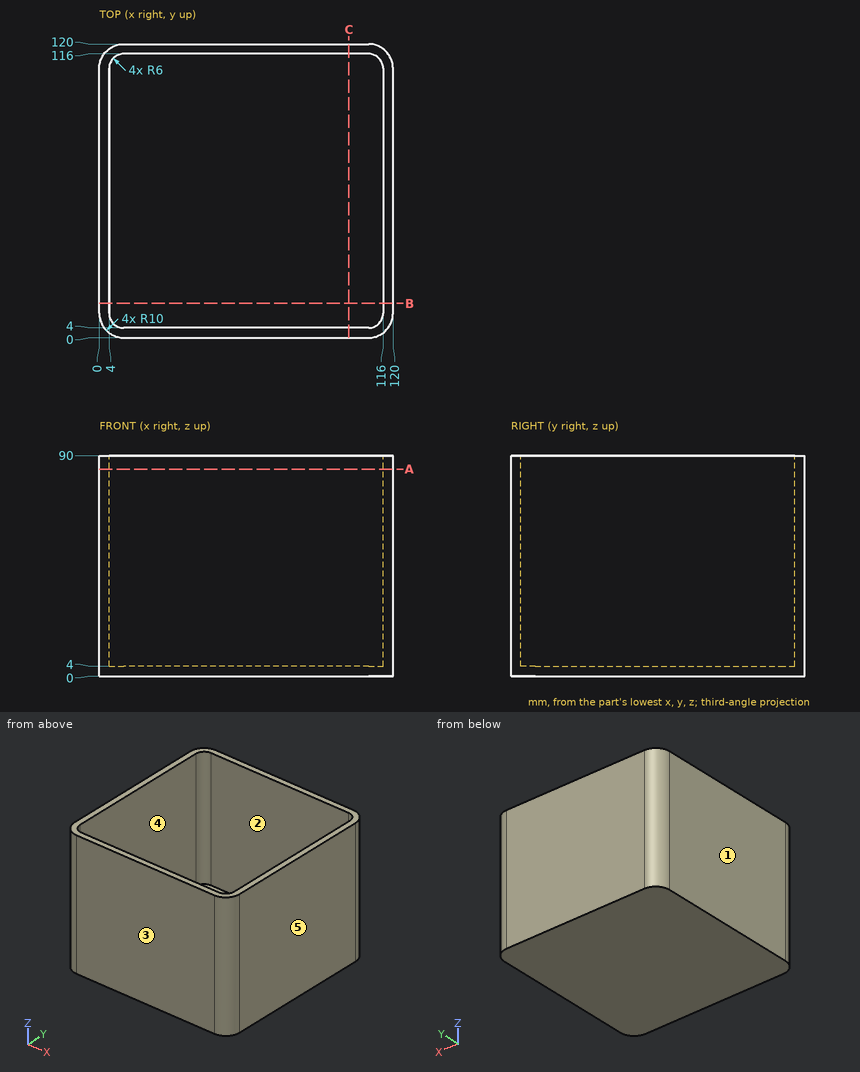
Answer from the drawing. Dimensions are ordinates in mm from the lowest x, y and z of the part. A direction names the side the tool comes from. Give positions to 0.01 mm unless a question says otherwise; leave off trailing zeros. Write each loop counter-clockwise with the first axis right and the second up, starting at its lowest first coordinate (ties: lowest second). Pieces come first, ordered by that corner, then holes. Notation, with made-up numbers: (-14.75, 59.25) - (19.25, 59.25) arc R27 cw to (19.25, 82.25) - close; hole circle Ø10 at (26.5, -39.75). An arc over 180 degrees is marked (long way). Answer in a Markdown table with one row per item. Add a question column.
Item 1: A flat-ended cylindrical pin translates along its axis: P1, Ø1.5, axis at x = 43, y = 78.5, coming from the +Z side. Find the tip coordinate at first contact, or state that the pin passes through.
Item 2: Section B-B, the plane y = 14 is taken. Write down the section's boundary in (x, z), and give its area (3 significant figures).
Item 3: Determine the mould class of the marked faces 3, 4 and 5 for opening direction Y: pulls with the +Y half, pulls with the -Y half, needs draft (parallel to the pull), parting line crosses it, or undercut.
Item 4: Find the intervals of material crossed by L1, parallel to Y at x = 99, z = 73; L2, parallel to Z at x = 106, y = 70.5, in increasing order.
Item 5: A tool of negligible diameter and unlimited length cuts with its end or side. For the marked faces 1 and 2, from which of +Z, -Z, +X, -X, +Y, -Y can it reach the whole face along a straight path? Write none if from no direction.
Item 6: Section A-A, the plane z = 84.5 is taken. Write down the section's boundary in (x, y).
Recorded:
| question | item | result |
|---|---|---|
| 1 | P1 | stops at z = 4 |
| 2 | outline | (0, 0) - (120, 0) - (120, 90) - (116, 90) - (116, 4) - (4, 4) - (4, 90) - (0, 90) - close |
| 2 | area | 1,170 mm2 |
| 3 | face 3 | pulls with the -Y half |
| 3 | face 4 | undercut |
| 3 | face 5 | needs draft |
| 4 | L1 | y = 0 to 4, 116 to 120 |
| 4 | L2 | z = 0 to 4 |
| 5 | face 1 | +Z, -Z, -X, +Y, -Y |
| 5 | face 2 | +Z |
| 6 | outline | (0, 10) arc R10 ccw to (10, 0) - (110, 0) arc R10 ccw to (120, 10) - (120, 110) arc R10 ccw to (110, 120) - (10, 120) arc R10 ccw to (0, 110) - close; hole (4, 10) arc R6 ccw to (10, 4) - (110, 4) arc R6 ccw to (116, 10) - (116, 110) arc R6 ccw to (110, 116) - (10, 116) arc R6 ccw to (4, 110) - close |
